```python
from build123d import *

# Parameters (mm, degrees)
BOSS_EXTRUDE1_DEPTH = 6
SKETCH2_R           = 1.1
CUT_EXTRUDE1_DEPTH  = 6
SKETCH3_R           = 1.1
CUT_EXTRUDE2_DEPTH  = 6


with BuildPart() as part:
    # Sketch1 → Boss-Extrude1 (new body)
    with BuildSketch(Plane.XY):
        Polygon((7.084804736, 1.368917583), (-2.915195264, 1.368917583), (-6.335396697, -8.028008625), (-4.456011456, -8.712048911), (-1.514780188, -0.631082417), (7.084804736, -0.631082417), align=None)
    extrude(amount=BOSS_EXTRUDE1_DEPTH)

    # Sketch2 → Cut-Extrude1 (cut)
    with BuildSketch(Plane(origin=(0, 1.368917583, 0), x_dir=(1, 0, 0), z_dir=(0, 1, 0))):
        with Locations(Location((4.084804736, -3, 0), (0, 0, 180))):
            Circle(SKETCH2_R)
    extrude(amount=-CUT_EXTRUDE1_DEPTH, mode=Mode.SUBTRACT)

    # Sketch3 → Cut-Extrude2 (cut)
    with BuildSketch(Plane(origin=(-3.014143829, 1.097058636, 0), x_dir=(0, 0, 1), z_dir=(-0.9396926207859095, 0.34202014332566544, 0))):
        with Locations(Location((3, -6.710693751, 0), (0, 0, 270))):
            Circle(SKETCH3_R)
    extrude(amount=-CUT_EXTRUDE2_DEPTH, mode=Mode.SUBTRACT)


solid = part.part
```
Work out the finished part from the listing and answer in its coordinate system (mm). Round coordinates to 2 decimals unless told otherwise and drop trailing zeros. Write each loop counter-clockwise with the first axis right and the second up, starting at its lowest first coordinate (ties: lowest second). Pieces come first, ordered by that corner, then holes.
1) A cutting plane is placed at C-C on y = 0.5. Determine the outline of the cut face in (x, z), and give its area (3 significant figures).
2) Consider probe 1 along Y at (x, z) = (2.5, 1.9); probe 2 along X at (y, z) = (-8, 5.45); probe 3 along X at (y, z) = (-1.25, 3.55). Determine where each line is inside the solid, lowest interval first.
3) Flat-ended cylindrical pins translate along their axes: P1, Ø1.5, axis at x = 1, y = -3, coming from the -Z side; P2, Ø1.5, axis at x = 1.5, z = 5, coming from the -Y side; P3, Ø1, axis at y = -1.5, z = 2.5, coming from the +X side; P4, Ø3, axis at y = -5, z = 2, coming from the +X side. Find the tip coordinate at first contact, or state that the pin passes through.
4) A cutting plane is placed at B-B on z = 3.4. Determine the outline of the cut face in (x, y).
5) Determine the mould class of faces 1 (the face through (-4.6, -3.26, 2.96)), 2 (the face through (7.085, 0, 3)), 3 (the face through (2.7, -0.631, 3)), 4 (the face through (-4.585, -6.102, 3.928)) for opening direction Y: pulls with the +Y half, pulls with the -Y half, needs draft (parallel to the pull), parting line crosses it, or undercut.
6) A cutting plane is placed at D-D on z = 5.25. Determine the outline of the cut face in (x, y), and give its area (3 significant figures).
7) A cutting plane is placed at A-A on x = 3.5. Determine the outline of the cut face in (y, z), and give its area (3 significant figures).
Entries:
1. outline: (-3.23, 0) - (7.08, 0) - (7.08, 6) - (-3.23, 6) - close; hole circle Ø2.2 at (4.08, 3)
1. area: 58.1 mm2
2. probe 1: y = -0.63 to 1.37
2. probe 2: x = -6.33 to -4.2
2. probe 3: x = -3.87 to -1.74
3. P1: passes through
3. P2: stops at y = -0.63
3. P3: stops at x = -1.65
3. P4: stops at x = -2.56
4. outline: (-6.34, -8.03) - (-4.46, -8.71) - (-3.78, -6.86) - (-5.66, -6.17) - close; (-4.96, -4.25) - (-3.08, -4.93) - (-1.51, -0.63) - (3.06, -0.63) - (3.06, 1.37) - (-2.92, 1.37) - close; (5.11, -0.63) - (7.08, -0.63) - (7.08, 1.37) - (5.11, 1.37) - close
5. face 1: pulls with the +Y half
5. face 2: needs draft
5. face 3: pulls with the -Y half
5. face 4: undercut
6. outline: (-6.34, -8.03) - (-4.46, -8.71) - (-1.51, -0.63) - (7.08, -0.63) - (7.08, 1.37) - (-2.92, 1.37) - close
6. area: 37.2 mm2
7. outline: (-0.63, 0) - (1.37, 0) - (1.37, 2.07) - (-0.63, 2.07) - close; (-0.63, 3.93) - (1.37, 3.93) - (1.37, 6) - (-0.63, 6) - close
7. area: 8.27 mm2
